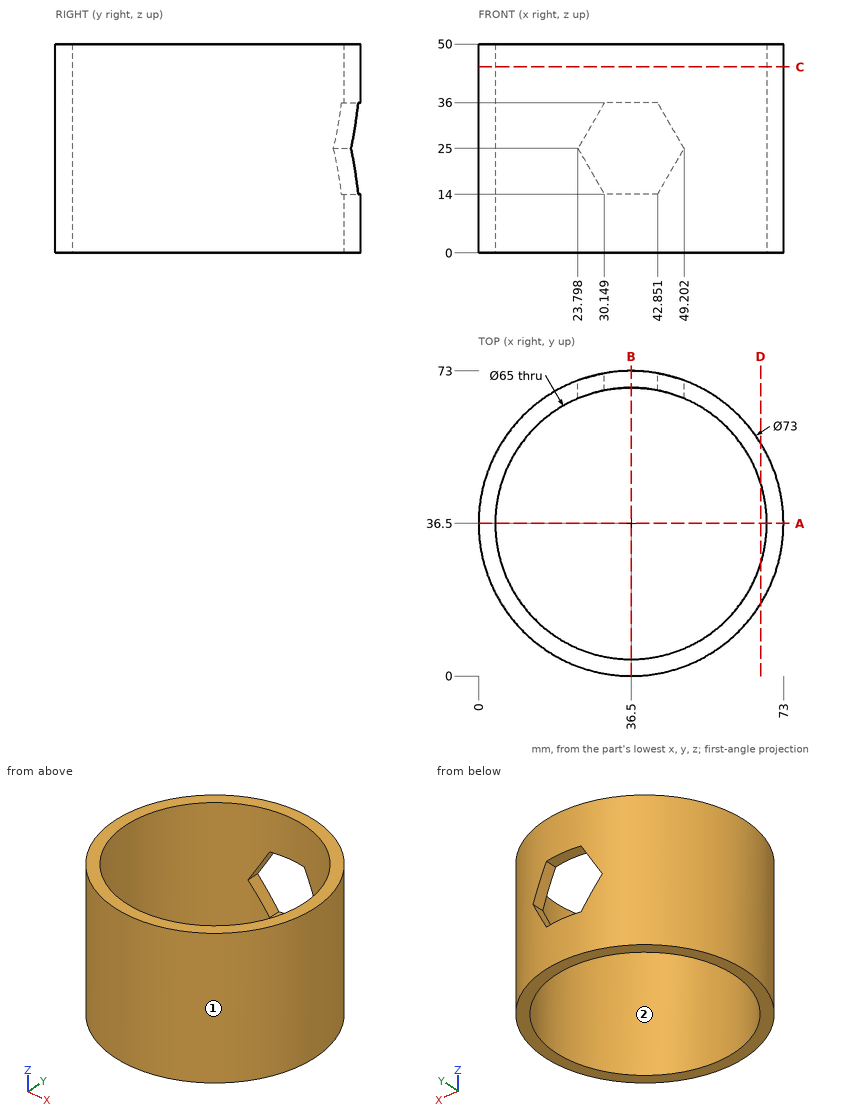
Job drawing, mm, ordinate dimensions from the low corner. One solid piece. Coordinates: 2 decimals unless noted, no trailing zeros. Order: outer loops, then holes, each group sorted by start corner. A loop starts at its lowest first (then second) coordinate and runs counter-clockwise, first axis right, second up. Notation, with made-up numbers: (9.25, 7) - (58.25, 7) arc R22 ccw to (58.25, 22) - close; hole circle Ø4 at (51.25, 58). An arc over 180 degrees is marked (long way). Return JSON: item names as keys, results as strings. Group by question number.
1) Saw through at D-D, the plane x = 67.5. Write the cut outline in (y, z), plus the area to 3 significant figures.
2) Saw through at A-A, the plane y = 36.5. Write the cut outline in (x, z).
3) Flat gauge pins, fed straight in: P1, Ø3, axis at y = 26, z = 16, coming from the -X side; P2, Ø1.4, axis at x = 37.5, y = 71.5, coming from the -Z side; P3, Ø10, axis at y = 29.5, z = 22, coming from the +X side (1 decimal); P4, Ø1, axis at y = 22, z = 18, coming from the -X side. Where does each tip first touch, or does it go through?
4) Mould opens along Y. For the marked faces 1 and 2 say: released by +Y, released by -Y, zero draft, split by the parting line, or undercut.
5) Saw through at C-C, the plane z = 44.5. Write the cut outline in (x, y).
6) Probe line 1 (X direction, y = 36, z = 26); line 2 (Y direction, x = 36, z = 20). List the from-to ranges inside material, lowest first. Write a range as from..to.
7) Saw through at B-B, the plane x = 36.5. Write the cut outline in (y, z).
Values found:
{
 "1": {"outline": "(17.23, 0) - (26.74, 0) - (26.74, 50) - (17.23, 50) - close; (46.26, 0) - (55.77, 0) - (55.77, 50) - (46.26, 50) - close", "area": "951 mm²"},
 "2": {"outline": "(0, 0) - (4, 0) - (4, 50) - (0, 50) - close; (69, 0) - (73, 0) - (73, 50) - (69, 50) - close"},
 "3": {"P1": "stops at x = 1.13", "P2": "stops at z = 0", "P3": "stops at x = 72.9", "P4": "stops at x = 2.79"},
 "4": {"face 1": "split by the parting line", "face 2": "undercut"},
 "5": {"outline": "circle Ø73 at (36.5, 36.5); hole circle Ø65 at (36.5, 36.5)"},
 "6": {"line 1": "x = 0..4, 69..73", "line 2": "y = 0..4"},
 "7": {"outline": "(0, 0) - (4, 0) - (4, 50) - (0, 50) - close; (69, 0) - (73, 0) - (73, 14) - (69, 14) - close; (69, 36) - (73, 36) - (73, 50) - (69, 50) - close"}
}
